Work out the finished part from the listing and answer in its coordinate system (mm). Face numbers are marked on the shaded views. A direction names the side the tool comes from. Coordinates: 2 decimals unless noted, no trailing zeros. Order: outer loops, then holes, each group sorted by start corner. A loop starts at its lowest first (then second) coordinate and runs counter-clockwise, first axis right, second up. Notation, with made-up numbers: (82, 86.5) - (121, 86.5) arc R18 cw to (121, 94.5) - close; hole circle Ø1 at (-5, 68.25). An arc over 180 degrees is marked (long way). Answer as a JSON object with one key per item and string values. Group by question number.
1) Find the intervals of material crossed by line 1 along Z through (x, y) = (12, 0.5); line 2 along X through (y, z) = (5.75, -18.9); line 3 along Z through (x, y) = (25, 1), in increasing order.
2) Section C-C (x = 41.5) is taken. Give the vertices of the cut face in (y, z).
3) Section B-B (z = -18.9) is taken. Give the vertices of the cut face in (x, y), plus the area to 3 significant figures.
4) A tool of negligible diameter and unlimited length cuts with its end or side. For the marked faces 1 and 2, from which of +Z, -Z, +X, -X, +Y, -Y can it reach the whole face along a straight path? Write none if from no direction.
5) Section D-D (y = 7.25) is taken. Give the vertices of the cut face in (x, z), plus the area to 3 significant figures.
6) Each of these flat-tipped pins is pushed along its axis until it touches: P1, Ø12, axis at x = 8, z = -8.5, coming from the +Y side; P2, Ø1.6, axis at y = 1, z = -18.5, coming from the +X side; P3, Ø2, axis at y = 6, z = -24, coming from the -X side. Where does it stop, or does it pass through?
7) Section A-A (x = 10.5) is taken. Give the vertices of the cut face in (y, z), plus the area to 3 significant figures.
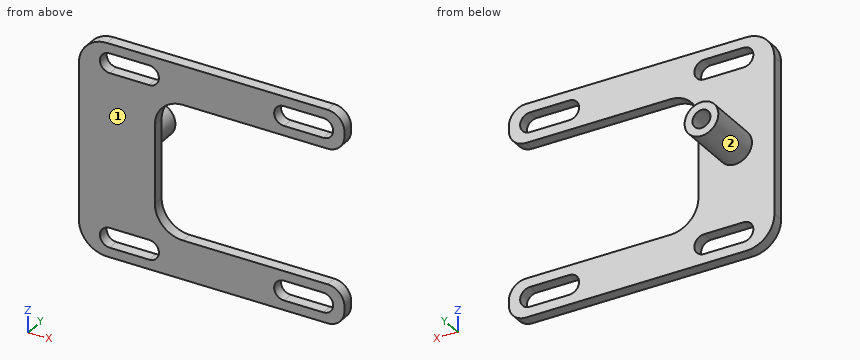
from build123d import *

# Parameters (mm, degrees)
BOSS_EXTRUDE1_DEPTH = 2
FILLET1_R           = 5
FILLET2_R           = 3
SKETCH2_R           = 3
SKETCH2_R_2         = 1.6
BOSS_EXTRUDE2_DEPTH = 10


with BuildPart() as part:
    # Sketch1 → Boss-Extrude1 (new body)
    with BuildSketch(Plane(origin=(0, 0, 0), x_dir=(1, 0, 0), z_dir=(0, 1, 0))):
        Polygon((47.24332582, 30.9), (47.24332582, 37.8), (0, 37.8), (0, 0), (47.24332582, 0), (47.24332582, 6.9), (13.518849419, 6.9), (13.518849419, 30.9), align=None)
        with BuildLine():
            Line((5.49332582, 36.1), (12.49332582, 36.1))
            ThreePointArc((12.49332582, 36.1), (14.24332582, 34.35), (12.49332582, 32.6))
            Line((12.49332582, 32.6), (5.49332582, 32.6))
            ThreePointArc((5.49332582, 32.6), (3.74332582, 34.35), (5.49332582, 36.1))
        make_face(mode=Mode.SUBTRACT)
        with BuildLine():
            Line((36.49332582, 36.1), (43.49332582, 36.1))
            ThreePointArc((43.49332582, 36.1), (45.24332582, 34.35), (43.49332582, 32.6))
            Line((43.49332582, 32.6), (36.49332582, 32.6))
            ThreePointArc((36.49332582, 32.6), (34.74332582, 34.35), (36.49332582, 36.1))
        make_face(mode=Mode.SUBTRACT)
        with BuildLine():
            Line((5.49332582, 5.2), (12.49332582, 5.2))
            ThreePointArc((12.49332582, 5.2), (14.24332582, 3.45), (12.49332582, 1.7))
            Line((12.49332582, 1.7), (5.49332582, 1.7))
            ThreePointArc((5.49332582, 1.7), (3.74332582, 3.45), (5.49332582, 5.2))
        make_face(mode=Mode.SUBTRACT)
        with BuildLine():
            Line((36.49332582, 5.2), (43.49332582, 5.2))
            ThreePointArc((43.49332582, 5.2), (45.24332582, 3.45), (43.49332582, 1.7))
            Line((43.49332582, 1.7), (36.49332582, 1.7))
            ThreePointArc((36.49332582, 1.7), (34.74332582, 3.45), (36.49332582, 5.2))
        make_face(mode=Mode.SUBTRACT)
    extrude(amount=BOSS_EXTRUDE1_DEPTH)

    # Fillet1
    fillet1_edges = [part.edges().sort_by_distance(p)[0] for p in [
        (13.518849419, 1, -6.9),
        (0, 1, 0),
        (0, 1, -37.8),
        (13.518849419, 1, -30.9),
    ]]
    fillet(fillet1_edges, radius=FILLET1_R)

    # Fillet2
    fillet2_edges = [part.edges().sort_by_distance(p)[0] for p in [
        (47.24332582, 1, -6.9),
        (47.24332582, 1, 0),
        (47.24332582, 1, -37.8),
        (47.24332582, 1, -30.9),
    ]]
    fillet(fillet2_edges, radius=FILLET2_R)

    # Sketch2 → Boss-Extrude2 (add)
    with BuildSketch(Plane(origin=(0, 2, 0), x_dir=(1, 0, 0), z_dir=(0, 1, 0))):
        with Locations(Location((6.99332582, 18.9, 0), (0, 0, 270))):
            Circle(SKETCH2_R)
        with Locations(Location((6.99332582, 18.9, 0), (0, 0, 270))):
            Circle(SKETCH2_R_2, mode=Mode.SUBTRACT)
    extrude(amount=BOSS_EXTRUDE2_DEPTH)


solid = part.part
Report:
{
 "1": {"line 1": "z = -37.8 to -36.1, -32.6 to -5.2, -1.7 to 0", "line 2": "x = 3.99 to 5.39, 8.59 to 9.99", "line 3": "z = -37.8 to -30.9, -6.9 to 0"},
 "2": {"outline": "(0, -37.8) - (2, -37.8) - (2, -36.1) - (0, -36.1) - close; (0, -32.6) - (2, -32.6) - (2, -30.9) - (0, -30.9) - close; (0, -6.9) - (2, -6.9) - (2, -5.2) - (0, -5.2) - close; (0, -1.7) - (2, -1.7) - (2, 0) - (0, 0) - close"},
 "3": {"outline": "(0, 0) - (13.52, 0) - (13.52, 2) - (9.99, 2) - (9.99, 12) - (8.59, 12) - (8.59, 2) - (5.39, 2) - (5.39, 12) - (3.99, 12) - (3.99, 2) - (0, 2) - close", "area": "55.0 mm²"},
 "4": {"face 1": "+Z, -Z, +X, -X, -Y", "face 2": "+Y"},
 "5": {"outline": "circle Ø6 at (6.99, -18.9); hole circle Ø3.2 at (6.99, -18.9)", "area": "20.2 mm²"},
 "6": {"P1": "stops at y = 2", "P2": "stops at x = 13.52", "P3": "passes through"},
 "7": {"outline": "(0, -37.8) - (2, -37.8) - (2, -36.1) - (0, -36.1) - close; (0, -32.6) - (2, -32.6) - (2, -5.2) - (0, -5.2) - close; (0, -1.7) - (2, -1.7) - (2, 0) - (0, 0) - close", "area": "61.6 mm²"}
}
